```python
from build123d import *

# Parameters (mm, degrees)
SKETCH1_W           = 102
SKETCH1_H           = 55
BOSS_EXTRUDE1_DEPTH = 131
SKETCH2_W           = 15.67927859
SKETCH2_H           = 4.373721057
SKETCH2_H_2         = 4.820111396
CUT_EXTRUDE1_DEPTH  = 2.54


with BuildPart() as part:
    # Sketch1 → Boss-Extrude1 (new body)
    with BuildSketch(Plane(origin=(0, 0, 0), x_dir=(1, 0, 0), z_dir=(0, 1, 0))):
        Rectangle(SKETCH1_W, SKETCH1_H)
    extrude(amount=BOSS_EXTRUDE1_DEPTH)

    # Sketch2 → Cut-Extrude1 (cut)
    # profile 1 of 7: a face of its own
    with BuildSketch(Plane.XY.offset(27.5)):
        with BuildLine():
            Line((32.222685011, 30.289063801), (16.543406421, 30.289063801))
            Line((16.543406421, 30.289063801), (16.543406421, 41.213310419))
            ThreePointArc((16.543406421, 41.213310419), (18.071687856, 44.464476673), (21.263986447, 46.112188983))
            Line((21.263986447, 46.112188983), (32.222685011, 46.112188983))
            Line((32.222685011, 46.112188983), (32.222685011, 41.796791207))
            Line((32.222685011, 41.796791207), (23.173438966, 41.796791207))
            ThreePointArc((23.173438966, 41.796791207), (21.378356157, 41.143325428), (20.571111013, 39.411940118))
            Line((20.571111013, 39.411940118), (20.571111013, 34.892154763))
            Line((20.571111013, 34.892154763), (32.222685011, 34.892154763))
            Line((32.222685011, 34.892154763), (32.222685011, 30.289063801))
        make_face()
    # profile 2 of 7: a face of its own
    with BuildSketch(Plane.XY.offset(27.5)):
        Polygon((32.222685011, 58.914535722), (32.222685011, 52.585285649), (16.543406421, 47.262961724), (16.543406421, 51.578359501), (29.001278605, 55.294208224), (16.543406421, 59.244665953), (16.543406421, 64.088679598), align=None)
    # profile 3 of 7: a face of its own
    with BuildSketch(Plane.XY.offset(27.5)):
        with Locations((24.383045716, 67.968593438)):
            Rectangle(SKETCH2_W, SKETCH2_H)
    # profile 4 of 7: a face of its own
    with BuildSketch(Plane.XY.offset(27.5)):
        with BuildLine():
            Line((32.222685011, 72.930180229), (16.543406421, 72.930180229))
            Line((16.543406421, 72.930180229), (16.543406421, 82.665236776))
            ThreePointArc((16.543406421, 82.665236776), (24.383045716, 88.291485928), (32.222685011, 82.665236776))
            Line((32.222685011, 82.665236776), (32.222685011, 72.930180229))
        make_face()
        with BuildLine():
            Line((20.335941045, 81.186975839), (20.335941045, 77.367606352))
            Line((20.335941045, 77.367606352), (29.001278605, 77.367606352))
            Line((29.001278605, 77.367606352), (29.001278605, 81.318517332))
            ThreePointArc((29.001278605, 81.318517332), (24.622917057, 84.262772166), (20.335941045, 81.186975839))
        make_face(mode=Mode.SUBTRACT)
    # profile 5 of 7: a face of its own
    with BuildSketch(Plane.XY.offset(27.5)):
        with Locations((24.383045716, 92.657631845)):
            Rectangle(SKETCH2_W, SKETCH2_H_2)
    # profile 6 of 7: a face of its own
    with BuildSketch(Plane.XY.offset(27.5)):
        Polygon((32.222685011, 96.757683119), (32.222685011, 101.073072233), (29.843242059, 101.863254429), (29.843242059, 109.239047859), (32.222685011, 110.484071773), (32.222685011, 115.184037049), (16.543406421, 108.92779188), (16.543406421, 102.796049103), align=None)
        Polygon((26.661750428, 108.457670817), (19.906160177, 105.955600354), (26.661750428, 103.153281435), align=None, mode=Mode.SUBTRACT)
    # profile 7 of 7: a face of its own
    with BuildSketch(Plane.XY.offset(27.5)):
        with BuildLine():
            Line((-6.115743329, 95.067687543), (-10.640576822, 87.427905373))
            ThreePointArc((-10.640576822, 87.427905373), (-1.813234505, 75.031176459), (0.903633442, 60.057216105))
            ThreePointArc((0.903633442, 60.057216105), (-4.465154431, 49.019149341), (-14.864068382, 42.497999922))
            ThreePointArc((-14.864068382, 42.497999922), (-21.425458539, 50.136520198), (-24.276421001, 59.794203453))
            ThreePointArc((-24.276421001, 59.794203453), (-22.06840901, 70.110226473), (-15.269017603, 78.17644767))
            ThreePointArc((-15.269017603, 78.17644767), (-9.151476423, 72.34247097), (-5.290820846, 64.822169595))
            ThreePointArc((-5.290820846, 64.822169595), (-5.118898357, 62.277928614), (-5.69667759, 59.794203453))
            ThreePointArc((-5.69667759, 59.794203453), (-8.801475151, 55.16826153), (-13.737803966, 52.585285649))
            ThreePointArc((-13.737803966, 52.585285649), (-16.38620677, 55.748861503), (-17.197044672, 59.794203453))
            ThreePointArc((-17.197044672, 59.794203453), (-15.016123652, 64.139522978), (-11.03158578, 66.925501483))
            Line((-11.03158578, 66.925501483), (-15.269017603, 72.262107708))
            ThreePointArc((-15.269017603, 72.262107708), (-19.465910752, 66.925501483), (-20.457305995, 60.20907285))
            ThreePointArc((-20.457305995, 60.20907285), (-18.493685046, 53.244585471), (-14.421821953, 47.262961724))
            ThreePointArc((-14.421821953, 47.262961724), (-6.68710858, 52.075713319), (-2.295755467, 60.057216105))
            ThreePointArc((-2.295755467, 60.057216105), (-5.69667759, 74.012425991), (-15.269380997, 84.721184263))
            ThreePointArc((-15.269380997, 84.721184263), (-24.537703565, 73.975429659), (-27.304719411, 60.057216105))
            ThreePointArc((-27.304719411, 60.057216105), (-23.293771998, 47.057349301), (-15.269380997, 36.07129518))
            ThreePointArc((-15.269380997, 36.07129518), (-2.295755467, 45.418962155), (4.139721094, 60.057216105))
            ThreePointArc((4.139721094, 60.057216105), (1.703886183, 78.350977538), (-6.115743329, 95.067687543))
        make_face()
    extrude(amount=-CUT_EXTRUDE1_DEPTH, mode=Mode.SUBTRACT)


solid = part.part
```
Input: part model. Units: mm. Frame: model coordinates. Give positions to 0.01 mm unless a question says otherwise; leave off trailing zeros. Return JSON: item names as keys, results as strings.
1) Mould query, pull axis X, two halves, no side actions, for faces 1 (the face through (24, 77, 24.96)), 2 (the face through (51, 65, 0)), 3 (the face through (-1, 0, 0)). Classes: released by +X, released by -X, zero draft, split by the parting line, or undercut.
Taken from the geometry:
{"face 1": "undercut", "face 2": "released by +X", "face 3": "zero draft"}
2) Contact query for a flat-ended pin moving along its axis: pin 1 (2 mm diameter, centred on x = 22.5, z = 26, fed in from -Y). Output: stop coordinate, or through.
Taken from the geometry:
{"pin 1": "stops at y = 0"}
3) Line query: L1, parallel to Z at x = -19, y = 81. Output: solid intervals per line, ascending. Write a range as [from, to].
Taken from the geometry:
{"L1": "z = [-27.5, 24.96]"}
